Could you check a few things on this drawing? It's one solid part, dimensions in mm from its lowest x, y, z. Round coordinates to 2 decimals unless told otherwise and drop trailing zeros. Loops run counter-clockwise (first coordinate to the right, second up) from the corner with the lowest first, then second, coordinate; pieces in that order, holes last. Notation, with made-up numbers: M 11,83 L 38,83 A19 cw 38,107 Z; hole C 83,82.25 d7. An arc over 180 degrees is marked long. Write item = value, one per line. Start each with the question number.
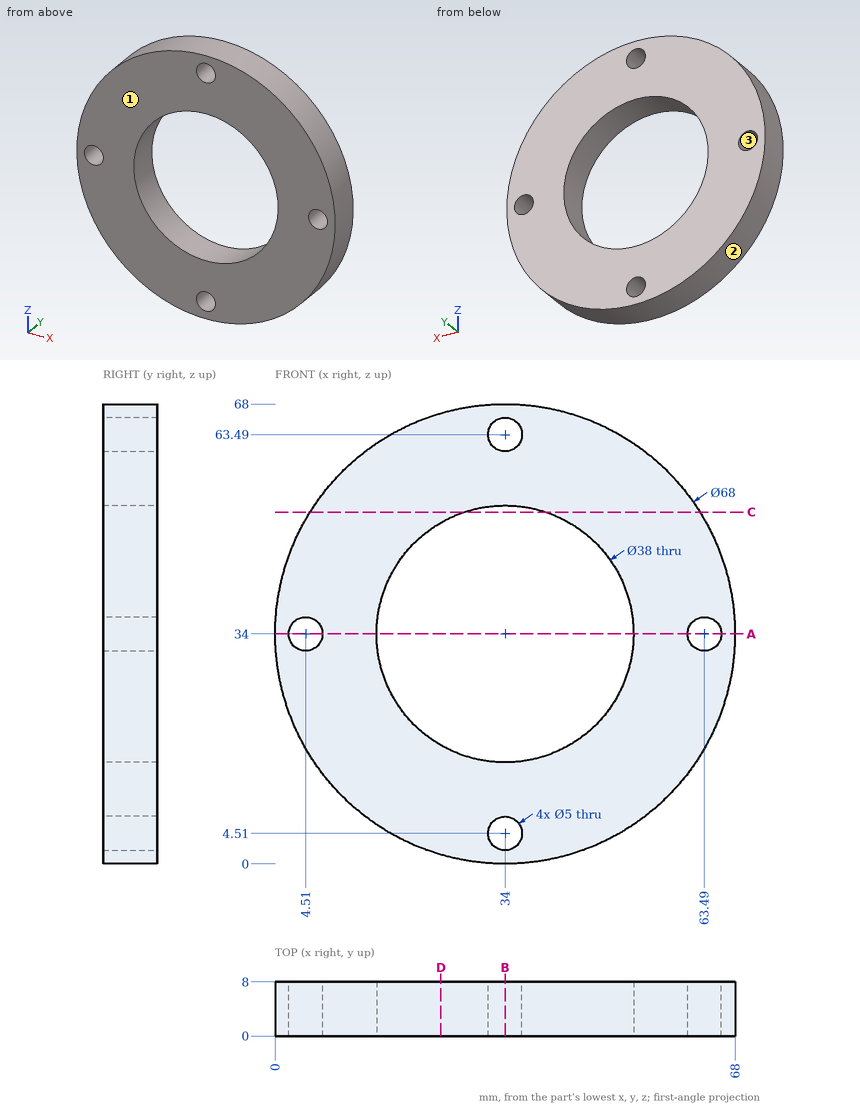
Item 1: Please list where these lines run through material, in increasing order: line 1 (X direction, y = 4.25, z = 34); line 2 (Z direction, x = 33, y = 1) (1 decimal); line 3 (Z direction, x = 32, y = 5.25) (1 decimal). Write a range as [from, to].
Item 2: I want a section at C-C, the plane z = 52. List the corners of the cut face in (x, y) for me (1 decimal).
Item 3: I want a section at D-D, the plane x = 24.5. List the corners of the cut face in (y, z) for me (1 decimal), then the cut area to 3 significant figures.
Item 4: I want a section at B-B, the plane x = 34. List the corners of the cut face in (y, z) for me, then the cut area to 3 significant figures.
Item 5: Will these pins go through, and if not, where does the flat tip stop? pin 1 Ø4 at (x, z) = (4.51, 34) entering from -Y; pin 2 Ø1.5 at (y, z) = (4.5, 46.5) entering from -X (1 decimal); pin 3 Ø1 at (x, y) = (35, 3.5) entering from -Z; pin 4 Ø3 at (x, y) = (32, 2.5) entering from +Z.
Item 6: We'd pull the mould along X, two halves only. Please class the marked faces 1, 2 and 3: released by +X, released by -X, zero draft, split by the parting line, or undercut.
Item 7: I want a section at A-A, the plane z = 34. List the corners of the cut face in (x, y) for me, then the cut area to 3 significant figures.
Worked out:
q1.line_1 = [0, 2.01], [7.01, 15], [53, 60.99], [65.99, 68]
q1.line_2 = [0, 2.2], [6.8, 15], [53, 61.2], [65.8, 68]
q1.line_3 = [0.1, 3], [6, 15.1], [52.9, 62], [65, 67.9]
q2.outline = M 5.2,0 L 27.9,0 L 27.9,8 L 5.2,8 Z; M 40.1,0 L 62.8,0 L 62.8,8 L 40.1,8 Z
q3.outline = M 0,1.4 L 8,1.4 L 8,17.5 L 0,17.5 Z; M 0,50.5 L 8,50.5 L 8,66.6 L 0,66.6 Z
q3.area = 259 mm2
q4.outline = M 0,0 L 8,0 L 8,2.01 L 0,2.01 Z; M 0,7.01 L 8,7.01 L 8,15 L 0,15 Z; M 0,53 L 8,53 L 8,60.99 L 0,60.99 Z; M 0,65.99 L 8,65.99 L 8,68 L 0,68 Z
q4.area = 160 mm2
q5.pin_1 = through
q5.pin_2 = 2.1
q5.pin_3 = 0
q5.pin_4 = 68
q6.face_1 = zero draft
q6.face_2 = split by the parting line
q6.face_3 = undercut
q7.outline = M 0,0 L 2.01,0 L 2.01,8 L 0,8 Z; M 7.01,0 L 15,0 L 15,8 L 7.01,8 Z; M 53,0 L 60.99,0 L 60.99,8 L 53,8 Z; M 65.99,0 L 68,0 L 68,8 L 65.99,8 Z
q7.area = 160 mm2
